Could you check a few things on this model? Use its own coordinates, in mm. Coordinates: 2 decimals unless noted, no trailing zeros. Use CSV: the item, a comma, the result in double quotes.
from build123d import *

# Parameters (mm, degrees)
CROQUIS1_R              = 4.1
SALIENTE_EXTRUIR1_DEPTH = 5
CROQUIS2_R              = 1.5
CORTAR_EXTRUIR1_DEPTH   = 10


with BuildPart() as part:
    # Croquis1 → Saliente-Extruir1 (new body)
    with BuildSketch(Plane(origin=(0, 0, 0), x_dir=(0, 1, 0), z_dir=(0, 0, 1))):
        with BuildLine():
            ThreePointArc((-72.5, 71.8), (-70.098275606, 77.598275606), (-64.3, 80))
            Line((-64.3, 80), (64.3, 80))
            ThreePointArc((64.3, 80), (70.098275606, 77.598275606), (72.5, 71.8))
            Line((72.5, 71.8), (72.5, -71.8))
            ThreePointArc((72.5, -71.8), (70.098275606, -77.598275606), (64.3, -80))
            Line((64.3, -80), (-64.3, -80))
            ThreePointArc((-64.3, -80), (-70.098275606, -77.598275606), (-72.5, -71.8))
            Line((-72.5, -71.8), (-72.5, 71.8))
        make_face()
        with Locations(Location((-64.3, -71.8, 0), (0, 0, 270))):
            Circle(CROQUIS1_R, mode=Mode.SUBTRACT)
        with Locations(Location((64.3, -71.8, 0), (0, 0, 270))):
            Circle(CROQUIS1_R, mode=Mode.SUBTRACT)
        with Locations(Location((64.3, 71.8, 0), (0, 0, 270))):
            Circle(CROQUIS1_R, mode=Mode.SUBTRACT)
        with Locations(Location((-64.3, 71.8, 0), (0, 0, 270))):
            Circle(CROQUIS1_R, mode=Mode.SUBTRACT)
    extrude(amount=SALIENTE_EXTRUIR1_DEPTH)

    # Croquis2 → Cortar-Extruir1 (cut)
    with BuildSketch(Plane(origin=(0, 0, 5), x_dir=(0, -1, 0), z_dir=(0, 0, 1))):
        with Locations(Location((-12.573190408, -41.986630744, 0), (0, 0, 90))):
            Circle(CROQUIS2_R)
        with Locations(Location((-12.618499373, 16.013437897, 0), (0, 0, 90))):
            Circle(CROQUIS2_R)
        with Locations(Location((36.241518275, 16.085874272, 0), (0, 0, 90))):
            Circle(CROQUIS2_R)
        with Locations(Location((36.426655653, -41.863805612, 0), (0, 0, 90))):
            Circle(CROQUIS2_R)
    extrude(amount=-CORTAR_EXTRUIR1_DEPTH, mode=Mode.SUBTRACT)


solid = part.part
(1) Please list where these lines run through material, in increasing order: line 1 (Y direction, x = -71.8, z = 3.9); line 2 (X direction, y = -37.5, z = 4.45); line 3 (X direction, y = -35.5, z = 3.5).
Computed:
line 1,"y = -72.5 to -68.4, -60.2 to 60.2, 68.4 to 72.5"
line 2,"x = -80 to -42.91, -40.82 to 15.27, 16.9 to 80"
line 3,"x = -80 to -43.04, -40.68 to 14.78, 17.39 to 80"
(2) Will this pin go through, and if not, where does the flat tip stop? pin 1 (2.5 mm diameter, centred on x = 16.09, y = -36.24, fed in from +Z).
Computed:
pin 1,"passes through"
(3) Thinking about a two-plate mould opening in Y: for faces 1 (the face through (80, 1, 2)), 2 (the face through (-77.662, 70.034, 2.465)), 3 (the face through (74, -60.84, 2.46)), which applies, +Y half, -Y half, draft (parallel to the pull), parting line (faces both ways), or undercut?
Computed:
face 1,"draft"
face 2,"+Y half"
face 3,"undercut"
